Read the model definition and answer for the solid it produces. Units are mm, in the model's axes. Face numbers are marked on the shaded views. A direction names the side the tool comes from. Give positions to 0.01 mm unless a question says otherwise; leave off trailing zeros. Loops run counter-clockwise (first coordinate to the right, second up) from the corner with the lowest first, then second, coordinate; pieces in that order, holes last. Notation, with made-up numbers: (-6, 39) -> (25, 39) arc R26 cw to (25, 58) -> close; hole circle Ø9 at (83, -11.75). An arc over 180 degrees is marked (long way). Answer as CSV lines item,"result". Start each with the question number.
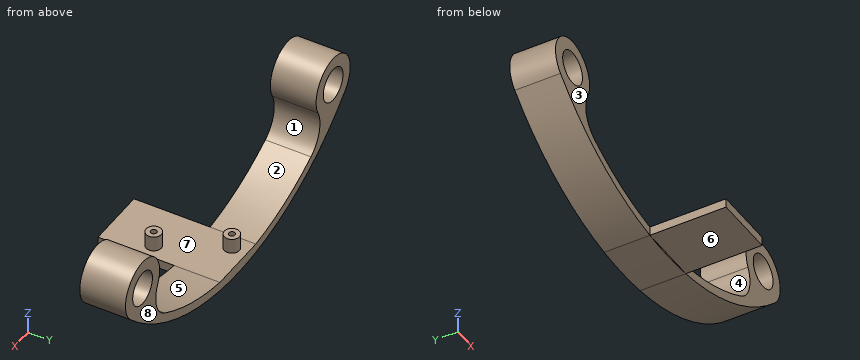
```python
from build123d import *

# Parameters (mm, degrees)
SKETCH1_W           = 20
SKETCH1_H           = 40
BOSS_EXTRUDE1_DEPTH = 3
SKETCH2_R           = 2.5
SKETCH2_R_2         = 1
BOSS_EXTRUDE2_DEPTH = 5
SKETCH3_R           = 5.5
BOSS_EXTRUDE3_DEPTH = 15


with BuildPart() as part:
    # Sketch1 → Boss-Extrude1 (new body)
    with BuildSketch(Plane.XY):
        with Locations((10, -20)):
            Rectangle(SKETCH1_W, SKETCH1_H)
    extrude(amount=BOSS_EXTRUDE1_DEPTH)

    # Sketch2 → Boss-Extrude2 (add)
    # profile 1 of 2: a face of its own
    with BuildSketch(Plane.XY.offset(3)):
        with Locations((4.83, -5)):
            Circle(SKETCH2_R)
        with Locations((4.83, -5)):
            Circle(SKETCH2_R_2, mode=Mode.SUBTRACT)
    # profile 2 of 2: a face of its own
    with BuildSketch(Plane.XY.offset(3)):
        with Locations((15.1678, -24.558)):
            Circle(SKETCH2_R)
        with Locations((15.1678, -24.558)):
            Circle(SKETCH2_R_2, mode=Mode.SUBTRACT)
    extrude(amount=BOSS_EXTRUDE2_DEPTH)

    # Sketch3 → Boss-Extrude3 (add)
    # profile 1 of 3: a face of its own
    with BuildSketch(Plane(origin=(0, 0, 0), x_dir=(1, 0, 0), z_dir=(0, 1, 0))):
        with BuildLine():
            Line((0, -3), (0, 0))
            ThreePointArc((0, 0), (-26.919603607, -7.898350205), (-49.769666667, -24.174824407))
            ThreePointArc((-49.769666667, -24.174824407), (-44.509522467, -40.277400292), (-34.608629413, -26.532059851))
            ThreePointArc((-34.608629413, -26.532059851), (-35.317872875, -19.127120719), (-30.717669917, -13.28124332))
            ThreePointArc((-30.717669917, -13.28124332), (-15.874630461, -6.599559407), (0, -3))
        make_face()
        with Locations(Location((-43.05, -30.890185893, 0), (0, 0, 270))):
            Circle(SKETCH3_R, mode=Mode.SUBTRACT)
    # profile 2 of 3: a face of its own
    with BuildSketch(Plane(origin=(0, 0, 0), x_dir=(1, 0, 0), z_dir=(0, 1, 0))):
        with BuildLine():
            ThreePointArc((69.769666667, -24.174824407), (46.919603607, -7.898350205), (20, 0))
            Line((20, 0), (20, -3))
            ThreePointArc((20, -3), (35.874630461, -6.599559407), (50.717669917, -13.28124332))
            ThreePointArc((50.717669917, -13.28124332), (55.317872875, -19.127120719), (54.608629413, -26.532059851))
            ThreePointArc((54.608629413, -26.532059851), (64.509522467, -40.277400292), (69.769666667, -24.174824407))
        make_face()
        with Locations(Location((63.05, -30.890185893, 0), (0, 0, 270))):
            Circle(SKETCH3_R, mode=Mode.SUBTRACT)
    # profile 3 of 3: a face of its own
    with BuildSketch(Plane(origin=(0, 0, 0), x_dir=(1, 0, 0), z_dir=(0, 1, 0))):
        with BuildLine():
            Line((0, 0), (20, 0))
            ThreePointArc((20, 0), (10, 0.593802374), (0, 0))
        make_face()
    extrude(amount=-BOSS_EXTRUDE3_DEPTH)


solid = part.part
```
(1) Find section D-D on y = -32.5. Write down the section's boundary in (x, z), then the cut area to 3 significant figures.
(2) The mould has two halves that part along X. Classify the marked faces 1, 2 and 3: pulls with the +X half, pulls with the -X half, needs draft (parallel to the pull), parting line crosses it, or undercut.
(3) Find section A-A on z = 18. Write down the section's boundary in (x, y).
(4) Find section C-C on y = -11. Write down the section's boundary in (x, z).
(5) A tool of negligible diameter and unlimited length cuts with its end or side. For the marked faces 4, 5, 6, 7 and 8, from which of +Z, -Z, +X, -X, +Y, -Y can it reach the whole face along a straight path? Write none if from no direction.
(6) Find the intervals of material crossed by line 1 along X through (y, z) = (-17, 2.5); line 2 along Z through (x, y) = (18.5, -18.5); line 3 along X through (y, z) = (-10, 14), in increasing order. Write a range as from..to.
(7) Each of these flat-tipped pins is pushed along its axis until it touches: P1, Ø4, axis at x = -37.5, z = 9.5, coming from the -Y side; P2, Ø3.5, axis at y = -27.5, z = 1.5, coming from the +X side; P3, Ø8, axis at y = -18, z = 33, coming from the -X side; P4, Ø1, axis at y = -25.5, z = 6.5, coming from the +X side. Where does it stop, or does it pass through?
(8) Find section B-B on x = -43.05. Write down the section's boundary in (y, z), then the cut area to 3 significant figures.
Answer block:
1,outline,"(0, 0) -> (20, 0) -> (20, 3) -> (0, 3) -> close"
1,area,"60.0 mm2"
2,face 1,"undercut"
2,face 2,"undercut"
2,face 3,"needs draft"
3,outline,"(-42.88, -15) -> (-34.91, -15) -> (-34.91, 0) -> (-42.88, 0) -> close; (54.91, -15) -> (62.88, -15) -> (62.88, 0) -> (54.91, 0) -> close"
4,outline,"(-49.77, 24.17) arc R84.5 ccw to (69.77, 24.17) arc R9.5 ccw (long way) to (54.61, 26.53) arc R10 cw to (50.72, 13.28) arc R81.52 cw to (20, 3) -> (0, 3) arc R81.52 cw to (-30.72, 13.28) arc R10 cw to (-34.61, 26.53) arc R9.5 ccw (long way) to start; hole circle Ø11 at (-43.05, 30.89); hole circle Ø11 at (63.05, 30.89)"
5,face 4,"+Y, -Y"
5,face 5,"+Z, +Y, -Y"
5,face 6,"-Z, +X, -X, -Y"
5,face 7,"+Z"
5,face 8,"+Z, -Z, +X, -X, +Y"
6,line 1,"x = 0..20"
6,line 2,"z = 0..3"
6,line 3,"x = -37.47..-31.8, 51.8..57.47"
7,P1,"passes through"
7,P2,"stops at x = 20"
7,P3,"stops at x = -52.55"
7,P4,"stops at x = 17.63"
8,outline,"(-15, 18.13) -> (0, 18.13) -> (0, 25.39) -> (-15, 25.39) -> close; (-15, 36.39) -> (0, 36.39) -> (0, 40.39) -> (-15, 40.39) -> close"
8,area,"169 mm2"
